Read the model definition and answer for the solid it produces. Units are mm, in the model's axes. A direction names the side the tool comes from. Coordinates: 2 decimals unless noted, no trailing zeros. Order: outer loops, then holes, each group sorted by start corner. A loop starts at its lowest first (then second) coordinate and runs counter-clockwise, first axis right, second up. Notation, with made-up numbers: (-5.5, 48.25) -> (38.5, 48.25) arc R21 cw to (38.5, 81.25) -> close; hole circle Ø6 at (-18, -24). An arc over 180 degrees is marked (long way). Answer as a JSON object with one key per item and string values. Group by question number.
1) Section D-D on y = 18 is taken. Determine the outline of the cut face in (x, z).
2) Section B-B on y = 43 is taken. Determine the outline of the cut face in (x, z).
3) Section C-C on x = 26.95 is taken. Determine the outline of the cut face in (y, z), and give its area (3 significant figures).
4) Given pin 1 (5 mm diameter, centred on x = 64, y = 4, fed in from +Z); pin 2 (0.8 mm diameter, centred on x = 10, z = -2.5, fed in from -Y); pin 3 (1 mm diameter, centred on y = 22.5, z = -5, fed in from -X); pin 4 (1 mm diameter, centred on x = 45.5, z = -2, fed in from -Y), each flat-ended and moving along its own axis, determine where each tip first touches the part or whether it passes through.
5) Consider L1, parallel to Y at x = 64, z = -6.15; L2, parallel to Y at x = 26.95, z = -1.35; L3, parallel to Y at x = 4, z = -6.45. Determine where each line is inside the solid, lowest interval first.
6) A tool of negligible diameter and unlimited length cuts with its end or side. For faces 1 (the cylindrical face through (4, 51, -2)), 2 (the flat face through (60, 43, -4)), 3 (the flat face through (34, 7, -3)), 4 (the flat face through (37.6, 7, -3)), from which of +Z, -Z, +X, -X, +Y, -Y can it reach the whole face along a straight path? Write none if from no direction.
7) Determine the mould class of faces 5 (the flat face through (27, 45, 0)), 6 (the cylindrical face through (10.4, 84.07, -5.42)), 7 (the cylindrical face through (56.633, 3.451, -2.697)) for opening direction Z: released by +Z, released by -Z, zero draft, split by the parting line, or undercut.
8) Section A-A on x = 53.3 is taken. Determine the outline of the cut face in (y, z).
from build123d import *

# Parameters (mm, degrees)
EXTRUDE_1_DEPTH          = 6
EXTRUDE_4_DEPTH          = 6.8
CUT_EXTRUDE_START        = -1.8
CUT_EXTRUDE_6_DEPTH      = 110.619208398
FILLET_1_R               = 2
CUT_EXTRUDE_4_DEPTH      = 112.419208398
CUT_EXTRUDE_4_DEPTH_BACK = 112.419208398
SKETCH_4_R               = 1.6
SKETCH_5_R               = 3.75
SKETCH_5_W               = 10.4
SKETCH_5_H               = 6.2
SKETCH_5_W_2             = 2.5
SKETCH_5_H_2             = 1
SKETCH_5_W_3             = 9.4
SKETCH_5_H_3             = 11.4
CUT_EXTRUDE_5_DEPTH      = 112.419208398
SKETCH_5_3_W             = 9.4
SKETCH_5_3_H             = 11.4
SKETCH_5_3_R             = 3.3
EXTRUDE_5_DEPTH          = 0.4
SKETCH_6_W               = 20
SKETCH_6_H               = 36
EXTRUDE_7_DEPTH          = 6
FILLET_2_R               = 2
FILLET_3_R               = 4
SKETCH_7_R               = 1.4
CUT_EXTRUDE_7_DEPTH      = 20
SKETCH_4_3_R             = 3
SKETCH_4_3_R_2           = 1.6
CUT_EXTRUDE_8_DEPTH      = 4
SKETCH_8_R               = 1.4
CUT_EXTRUDE_9_DEPTH      = 7
CHAMFER_1_SIZE           = 1.4


with BuildPart() as part:
    # 草图1 → 凸台-拉伸1 (new body)
    with BuildSketch(Plane.XY):
        Polygon((0, 0), (68, 0), (68, 88), (8, 88), (8, 52), (0, 52), align=None)
    extrude(amount=-EXTRUDE_1_DEPTH)

    # 草图1<2> → 凸台-拉伸4 (add)
    with BuildSketch(Plane.XY):
        Polygon((2.2, 49.8), (2.2, 2.2), (65.8, 2.2), (65.8, 85.8), (10.2, 85.8), (10.2, 49.8), align=None)
        Polygon((8, 44), (8, 8), (60, 8), (60, 80), (16, 80), (16, 44), align=None, mode=Mode.SUBTRACT)
    extrude(amount=-EXTRUDE_4_DEPTH)

    # 草图1<5> → 切除-拉伸6 (cut, through all)
    with BuildSketch(Plane.XY.offset(CUT_EXTRUDE_START)):
        Polygon((16, 80), (16, 44), (8, 44), (8, 8), (60, 8), (60, 80), align=None)
    extrude(amount=-CUT_EXTRUDE_6_DEPTH, mode=Mode.SUBTRACT)

    # 圆角1
    fillet_1_edges = [part.edges().sort_by_distance(p)[0] for p in [
        (68, 88, -3),
        (68, 0, -3),
        (0, 0, -3),
        (10.2, 85.8, -6.4),
        (65.8, 85.8, -6.4),
        (65.8, 2.2, -6.4),
        (2.2, 2.2, -6.4),
        (2.2, 49.8, -6.4),
    ]]
    fillet(fillet_1_edges, radius=FILLET_1_R)

    # 草图4 → 切除-拉伸4 (cut, two sides: drawn at the far end of the back side and taken through both)
    with BuildSketch(Plane.XY.offset(-CUT_EXTRUDE_4_DEPTH_BACK)):
        with Locations((12, 84)):
            Circle(SKETCH_4_R)
        with Locations((64, 84)):
            Circle(SKETCH_4_R)
        with Locations((64, 4)):
            Circle(SKETCH_4_R)
        with Locations((4, 48)):
            Circle(SKETCH_4_R)
        with Locations((4, 4)):
            Circle(SKETCH_4_R)
        with Locations((64, 48)):
            Circle(SKETCH_4_R)
    extrude(amount=CUT_EXTRUDE_4_DEPTH + CUT_EXTRUDE_4_DEPTH_BACK, mode=Mode.SUBTRACT)

    # 草图5 → 切除-拉伸5 (cut, through all)
    with BuildSketch(Plane.XY):
        with Locations((26.95, 20.7)):
            Circle(SKETCH_5_R)
        with Locations((42.8, 8.3)):
            Rectangle(SKETCH_5_W, SKETCH_5_H)
        with Locations((26.95, 14.7)):
            Rectangle(SKETCH_5_W_2, SKETCH_5_H_2)
        with Locations((53.3, 18.1)):
            Rectangle(SKETCH_5_W_3, SKETCH_5_H_3)
    extrude(amount=-CUT_EXTRUDE_5_DEPTH, mode=Mode.SUBTRACT)

    # 草图5<3> → 凸台-拉伸5 (add)
    with BuildSketch(Plane.XY):
        with Locations((53.3, 18.1)):
            Rectangle(SKETCH_5_3_W, SKETCH_5_3_H)
        with Locations((53.3, 19)):
            Circle(SKETCH_5_3_R, mode=Mode.SUBTRACT)
    extrude(amount=-EXTRUDE_5_DEPTH)

    # 草图6 → 凸台-拉伸7 (add)
    with BuildSketch(Plane.XY):
        with Locations((-2, 70)):
            Rectangle(SKETCH_6_W, SKETCH_6_H)
    extrude(amount=-EXTRUDE_7_DEPTH)

    # 圆角2
    fillet_2_edges = [part.edges().sort_by_distance(p)[0] for p in [
        (0, 52, -3),
    ]]
    fillet(fillet_2_edges, radius=FILLET_2_R)

    # 圆角3
    fillet_3_edges = [part.edges().sort_by_distance(p)[0] for p in [
        (-12, 52, -3),
    ]]
    fillet(fillet_3_edges, radius=FILLET_3_R)

    # 草图7 → 切除-拉伸7 (cut)
    with BuildSketch(Plane.ZY.offset(12)):
        with Locations((-3, 82)):
            Circle(SKETCH_7_R)
        with Locations((-3, 62)):
            Circle(SKETCH_7_R)
    extrude(amount=-CUT_EXTRUDE_7_DEPTH, mode=Mode.SUBTRACT)

    # 草图4<3> → 切除-拉伸8 (cut)
    # profile 1 of 6: a face of its own
    with BuildSketch(Plane.XY):
        with Locations((12, 84)):
            Circle(SKETCH_4_3_R)
        with Locations((12, 84)):
            Circle(SKETCH_4_3_R_2, mode=Mode.SUBTRACT)
    # profile 2 of 6: a face of its own
    with BuildSketch(Plane.XY):
        with Locations((64, 84)):
            Circle(SKETCH_4_3_R)
        with Locations((64, 84)):
            Circle(SKETCH_4_3_R_2, mode=Mode.SUBTRACT)
    # profile 3 of 6: a face of its own
    with BuildSketch(Plane.XY):
        with Locations((4, 48)):
            Circle(SKETCH_4_3_R)
        with Locations((4, 48)):
            Circle(SKETCH_4_3_R_2, mode=Mode.SUBTRACT)
    # profile 4 of 6: a face of its own
    with BuildSketch(Plane.XY):
        with Locations((64, 48)):
            Circle(SKETCH_4_3_R)
        with Locations((64, 48)):
            Circle(SKETCH_4_3_R_2, mode=Mode.SUBTRACT)
    # profile 5 of 6: a face of its own
    with BuildSketch(Plane.XY):
        with Locations((4, 4)):
            Circle(SKETCH_4_3_R)
        with Locations((4, 4)):
            Circle(SKETCH_4_3_R_2, mode=Mode.SUBTRACT)
    # profile 6 of 6: a face of its own
    with BuildSketch(Plane.XY):
        with Locations((64, 4)):
            Circle(SKETCH_4_3_R)
        with Locations((64, 4)):
            Circle(SKETCH_4_3_R_2, mode=Mode.SUBTRACT)
    extrude(amount=-CUT_EXTRUDE_8_DEPTH, mode=Mode.SUBTRACT)

    # 草图8 → 切除-拉伸9 (cut)
    with BuildSketch(Plane.XZ):
        with Locations(Location((58, -3, 0), (0, 0, 270))):
            Circle(SKETCH_8_R)
        with Locations(Location((10, -3, 0), (0, 0, 270))):
            Circle(SKETCH_8_R)
        with Locations(Location((34, -3, 0), (0, 0, 270))):
            Circle(SKETCH_8_R)
    extrude(amount=-CUT_EXTRUDE_9_DEPTH, mode=Mode.SUBTRACT)

    # 倒角1
    chamfer_1_edges = [part.edges().sort_by_distance(p)[0] for p in [
        (2.4, 4, -4),
        (62.4, 48, -4),
        (2.4, 48, -4),
        (62.4, 84, -4),
        (62.4, 4, -4),
        (9, 84, -4),
    ]]
    chamfer(chamfer_1_edges, length=CHAMFER_1_SIZE - 0.0001)  # a hair under: the kernel refuses the full size


solid = part.part
Worked answers:
{
 "1": {"outline": "(0, -6) -> (2.2, -6) -> (2.2, -6.8) -> (8, -6.8) -> (8, -1.8) -> (24.35, -1.8) -> (24.35, 0) -> (0, 0) -> close; (29.55, -1.8) -> (48.6, -1.8) -> (48.6, -0.4) -> (50.16, -0.4) -> (50.16, 0) -> (29.55, 0) -> close; (56.44, -0.4) -> (58, -0.4) -> (58, -1.8) -> (60, -1.8) -> (60, -6.8) -> (65.8, -6.8) -> (65.8, -6) -> (68, -6) -> (68, 0) -> (56.44, 0) -> close"},
 "2": {"outline": "(0, -6) -> (2.2, -6) -> (2.2, -6.8) -> (8, -6.8) -> (8, -1.8) -> (60, -1.8) -> (60, -6.8) -> (65.8, -6.8) -> (65.8, -6) -> (68, -6) -> (68, 0) -> (0, 0) -> close"},
 "3": {"outline": "(0, -6) -> (2.2, -6) -> (2.2, -6.8) -> (8, -6.8) -> (8, -1.8) -> (14.2, -1.8) -> (14.2, 0) -> (0, 0) -> close; (15.2, -1.8) -> (16.95, -1.8) -> (16.95, 0) -> (15.2, 0) -> close; (24.45, -1.8) -> (80, -1.8) -> (80, -6.8) -> (85.8, -6.8) -> (85.8, -6) -> (88, -6) -> (88, 0) -> (24.45, 0) -> close", "area": "220 mm²"},
 "4": {"pin 1": "stops at z = -4.5", "pin 2": "stops at y = 7", "pin 3": "stops at x = 0", "pin 4": "stops at y = 0"},
 "5": {"L1": "y = 2.21 to 2.4, 5.6 to 46.4, 49.6 to 82.4, 85.6 to 85.79", "L2": "y = 0 to 14.2, 15.2 to 16.95, 24.45 to 88", "L3": "y = 2.21 to 2.4, 5.6 to 46.4, 49.6 to 49.79"},
 "6": {"face 1": "+Z", "face 2": "-Z", "face 3": "-Y", "face 4": "+Z, -Z"},
 "7": {"face 5": "released by +Z", "face 6": "zero draft", "face 7": "undercut"},
 "8": {"outline": "(0, -6) -> (2.2, -6) -> (2.2, -6.8) -> (8, -6.8) -> (8, -1.8) -> (12.4, -1.8) -> (12.4, -0.4) -> (15.7, -0.4) -> (15.7, 0) -> (0, 0) -> close; (22.3, -0.4) -> (23.8, -0.4) -> (23.8, -1.8) -> (80, -1.8) -> (80, -6.8) -> (85.8, -6.8) -> (85.8, -6) -> (88, -6) -> (88, 0) -> (22.3, 0) -> close"}
}
